Could you check a few things on this model? Use its own coordinates, in mm. Coordinates: 2 decimals unless noted, no trailing zeros. Loops run counter-clockwise (first coordinate to the right, second up) from the corner with the lowest first, then second, coordinate; pieces in that order, holes last.
from build123d import *

# Parameters (mm, degrees)
SKETCH1_W            = 110
SKETCH1_H            = 20
BOSS_EXTRUDE1_DEPTH  = 2.5
M3_CLEARANCE_HOLE1_D = 3.4


with BuildPart() as part:
    # Sketch1 → Boss-Extrude1 (new, symmetric)
    with BuildSketch(Plane(origin=(0, 0, 0), x_dir=(1, 0, 0), z_dir=(0, 1, 0))):
        Rectangle(SKETCH1_W, SKETCH1_H)
    extrude(amount=BOSS_EXTRUDE1_DEPTH, both=True)

    # M3 Clearance Hole1 (through all)
    with Locations(Plane(origin=(0, 2.5, 0), x_dir=(1, 0, 0), z_dir=(0, 1, 0))):
        with Locations((-17.275, 0), (-51.825, -6), (51.825, -6), (-51.825, 6), (51.825, 6), (17.275, 0)):
            Hole(M3_CLEARANCE_HOLE1_D / 2)


solid = part.part
(1) We'd pull the mould along Z, two halves only. Please class faces 1 (the face through (-55, 0, 0)), 2 (the face through (-1, 0, 10)), 3 (the face through (-50.127, -0.035, 5.925)): +Z half, -Z half, draft (parallel to the pull), parting line (faces both ways), or undercut.
Answers:
face 1: draft
face 2: +Z half
face 3: undercut
(2) I need wall thicknesses on probe 1 along X at (y, z) = (0.8, -6) (3 decimals); probe 2 along Z at (x, y) = (50.5, 1.65); probe 3 along X at (y, z) = (1.45, 7.25). Which ranges of each line are inside material? Lowest first, please.
Answers:
probe 1: x = -55 to -53.525, -50.125 to 50.125, 53.525 to 55
probe 2: z = -10 to -7.07, -4.93 to 4.93, 7.07 to 10
probe 3: x = -55 to -52.98, -50.67 to 50.67, 52.98 to 55
(3) Imagine slicing it at B-B, the plane y = -0.3. Write out the boundary of the cut face in (x, z) (3 decimals), and give its area (3 significant figures).
Answers:
outline: (-55, -10) - (55, -10) - (55, 10) - (-55, 10) - close; hole circle Ø3.4 at (-51.825, -6); hole circle Ø3.4 at (-51.825, 6); hole circle Ø3.4 at (-17.275, 0); hole circle Ø3.4 at (17.275, 0); hole circle Ø3.4 at (51.825, -6); hole circle Ø3.4 at (51.825, 6)
area: 2,150 mm2
(4) Imagine slicing it at A-A, the plane z = -6. Write out the boundary of the cut face in (x, y) (3 decimals).
Answers:
outline: (-55, -2.5) - (-53.525, -2.5) - (-53.525, 2.5) - (-55, 2.5) - close; (-50.125, -2.5) - (50.125, -2.5) - (50.125, 2.5) - (-50.125, 2.5) - close; (53.525, -2.5) - (55, -2.5) - (55, 2.5) - (53.525, 2.5) - close
